The listing builds one solid part. Answer for the finished solid, in the listing's coordinates (mm). Face numbers are marked on the shaded views. A direction names the side the tool comes from. Give positions to 0.01 mm unless a question says otherwise; leave off trailing zeros. Order: outer loops, then holes, each group sorted by start corner. A loop starts at its lowest first (then second) coordinate and runs counter-clockwise, first axis right, second up. Notation, with made-up numbers: (79.25, 85.25) - (121.25, 85.25) arc R28 cw to (121.25, 115.25) - close; hole circle Ø8 at (-2.75, 42). An arc over 180 degrees is marked (long way). Write each question's results on one line, items separated by ' | '. Start each with the question number.
1. Flat-ended cylindrical pins translate along their axes: pin 1 (1 mm diameter, centred on x = 15.88, z = 12.38, fed in from -Y); pin 2 (1.8 mm diameter, centred on x = -15.875, z = 10, fed in from -Y); pin 3 (0.6 mm diameter, centred on y = 3.5, z = -17.5, fed in from +X); pin 4 (2 mm diameter, centred on x = -15.88, z = 5.22, fed in from +Y). Find the tip coordinate at first contact, or state that the pin passes through.
2. Section A-A (z = 10) is taken. Give the vertices of the cut face in (x, y).
3. Determine the mould class of the marked faces 4 and 5 for opening direction Z: released by +Z, released by -Z, zero draft, split by the parting line, or undercut.
4. Find the intervals of material crossed by L1, parallel to X at y = 2, z = 5; L2, parallel to X at y = 0.5, z = 16; L3, parallel to Y at x = 5, z = -12.5, in increasing order.
5. Which of the six approach directions +Z, -Z, +X, -X, +Y, -Y give full straight-line access (tool end or side, diameter ignored) to the marked faces 1, 2 and 3?
6. Section C-C (x = -14) is taken. Give the vertices of the cut face in (y, z).
7. Section B-B (y = 3) is taken. State how many separate pieces and enclosed holes the cut face has, and give its area (3 significant figures).
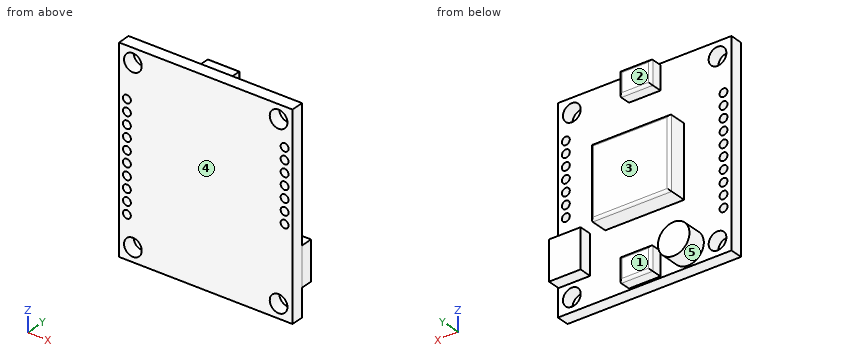
from build123d import *

# Parameters (mm, degrees)
SKETCH1_W                           = 34.925
SKETCH1_H                           = 40
BOSS_EXTRUDE1_DEPTH                 = 2.54
F_9_64_0_14063_DIAMETER_HOLE1_D     = 3.572002
F_9_64_0_14063_DIAMETER_HOLE1_DEPTH = 2.54
F_1_16_0_0625_DIAMETER_HOLE1_D      = 1.5875
F_1_16_0_0625_DIAMETER_HOLE1_DEPTH  = 2.54
SKETCH6_R                           = 3.175
BOSS_EXTRUDE2_DEPTH                 = 3.81
SKETCH7_W                           = 15.875
SKETCH7_H                           = 14.2875
BOSS_EXTRUDE3_DEPTH                 = 3.81
FILLET1_R                           = 0.508
SKETCH8_W                           = 6.35
SKETCH8_H                           = 7.874
BOSS_EXTRUDE4_DEPTH                 = 2.54
SKETCH10_W                          = 6.35
SKETCH10_H                          = 4.7625
BOSS_EXTRUDE5_DEPTH                 = 2.54
FILLET2_R                           = 0.508


with BuildPart() as part:
    # Sketch1 → Boss-Extrude1 (new body)
    with BuildSketch(Plane(origin=(0, 0, 0), x_dir=(1, 0, 0), z_dir=(0, 1, 0))):
        Rectangle(SKETCH1_W, SKETCH1_H)
    extrude(amount=BOSS_EXTRUDE1_DEPTH)

    # 9/64 (0.14063) Diameter Hole1
    with Locations(Plane(origin=(0, 2.54, 0), x_dir=(1, 0, 0), z_dir=(0, 1, 0))):
        with Locations((-14.6685, 17.206), (14.6685, 17.206), (14.6685, -17.206), (-14.6685, -17.206)):
            Hole(F_9_64_0_14063_DIAMETER_HOLE1_D / 2, depth=F_9_64_0_14063_DIAMETER_HOLE1_DEPTH)

    # 1/16 (0.0625) Diameter Hole1
    with Locations(Plane(origin=(0, 2.54, 0), x_dir=(1, 0, 0), z_dir=(0, 1, 0))):
        with Locations((-15.875, -10), (-15.875, -7.6124), (-15.875, -5.2248), (-15.875, -2.8372), (-15.875, -0.4496), (-15.875, 1.938), (-15.875, 4.3256), (-15.875, 6.7132), (-15.875, 9.1008), (-15.875, 11.4884), (15.875, 1.938), (15.875, -0.4496), (15.875, -2.8372), (15.875, -5.2248), (15.875, -7.6124), (15.875, -10), (15.875, -12.38125)):
            Hole(F_1_16_0_0625_DIAMETER_HOLE1_D / 2, depth=F_1_16_0_0625_DIAMETER_HOLE1_DEPTH)

    # Sketch6 → Boss-Extrude2 (add)
    with BuildSketch(Plane(origin=(0, 2.54, 0), x_dir=(1, 0, 0), z_dir=(0, 1, 0))):
        with Locations((-8.73125, 16.5125)):
            Circle(SKETCH6_R)
    extrude(amount=BOSS_EXTRUDE2_DEPTH)

    # Sketch7 → Boss-Extrude3 (add)
    with BuildSketch(Plane(origin=(0, 2.54, 0), x_dir=(1, 0, 0), z_dir=(0, 1, 0))):
        Rectangle(SKETCH7_W, SKETCH7_H)
    extrude(amount=BOSS_EXTRUDE3_DEPTH)

    # Fillet1
    fillet1_edges = [part.edges().sort_by_distance(p)[0] for p in [
        (7.9375, 6.35, 0),
        (0, 6.35, -7.14375),
        (-7.9375, 6.35, 0),
        (0, 6.35, 7.14375),
    ]]
    fillet(fillet1_edges, radius=FILLET1_R)

    # Sketch8 → Boss-Extrude4 (add)
    with BuildSketch(Plane(origin=(0, 2.54, 0), x_dir=(1, 0, 0), z_dir=(0, 1, 0))):
        with Locations((14.1605, 10.607)):
            Rectangle(SKETCH8_W, SKETCH8_H)
    extrude(amount=BOSS_EXTRUDE4_DEPTH)

    # Sketch10 → Boss-Extrude5 (add)
    with BuildSketch(Plane(origin=(0, 2.54, 0), x_dir=(1, 0, 0), z_dir=(0, 1, 0))):
        with Locations((-0.010133196, 17.333)):
            Rectangle(SKETCH10_W, SKETCH10_H)
        with Locations((-0.010133196, -17.333)):
            Rectangle(SKETCH10_W, SKETCH10_H)
    extrude(amount=BOSS_EXTRUDE5_DEPTH)

    # Fillet2
    fillet2_edges = [part.edges().sort_by_distance(p)[0] for p in [
        (-3.185133196, 5.08, -17.333),
        (-0.010133196, 5.08, -14.95175),
        (3.164866804, 5.08, -17.333),
        (-0.010133196, 5.08, -19.71425),
        (3.164866804, 5.08, 17.333),
        (-0.010133196, 5.08, 14.95175),
        (-3.185133196, 5.08, 17.333),
        (-0.010133196, 5.08, 19.71425),
    ]]
    fillet(fillet2_edges, radius=FILLET2_R)


solid = part.part
Reported:
1) pin 1: through | pin 2: y = 0 | pin 3: x = 3.16 | pin 4: y = 2.54
2) outline: (-17.46, 0) - (-16.67, 0) - (-16.67, 2.54) - (-17.46, 2.54) - close; (-15.08, 0) - (15.08, 0) - (15.08, 2.54) - (-15.08, 2.54) - close; (16.67, 0) - (17.46, 0) - (17.46, 2.54) - (16.67, 2.54) - close
3) face 4: zero draft | face 5: undercut
4) L1: -17.46 to -16.64, -15.11 to 15.11, 16.64 to 17.46 | L2: -17.46 to -15.99, -13.35 to 13.35, 15.99 to 17.46 | L3: 0 to 2.54
5) face 1: -Z, +X, +Y | face 2: +Z, +X, -X, +Y | face 3: +Z, -Z, +X, -X, +Y
6) outline: (0, -20) - (2.54, -20) - (2.54, -18.86) - (0, -18.86) - close; (0, -15.55) - (2.54, -15.55) - (2.54, 15.55) - (0, 15.55) - close; (0, 18.86) - (2.54, 18.86) - (2.54, 20) - (0, 20) - close
7) separate pieces: 5 | enclosed holes: 0 | area: 369 mm²
